Geometry check sheet. Reference: drawing and pictorial views, mm from the part's lowest x, y, z. Round coordinates to 2 decimals unless told otherwise and drop trailing zeros. Loops run counter-clockwise (first coordinate to the right, second up) from the corner with the lowest first, then second, coordinate; pieces in that order, holes last. Notation, with made-up numbers: (22, -19.5) -> (48, -19.5) arc R33 ccw to (48, 14.5) -> close; hole circle Ø8 at (16, 51). An arc over 180 degrees is marked (long way). Use one line per item in the form item = value. Start each with the question number.
(1) Material ranges on probe 1 along Y at (x, z) = (150, 17.75); probe 2 along X at (y, z) = (51.5, 20.75); probe 3 along X at (y, z) = (33.5, 17), recorded low to high. Write a range as [from, to].
(2) Sectioned sample at A-A (y = 50). Record the cut outline in (x, z), and give its area (3 significant figures).
(3) Draft check along X on the marked faces 1, 2 and 3. Enter one of: released by +X, released by -X, zero draft, split by the parting line, or undercut.
(4) Go/stop test with a flat-tipped pin: pin 1 (1 mm diameter, centred on y = 88, z = 22.5, fed in from -X). Record where the tip stops, or that it passes through.
(5) Sectioned sample at C-C (z = 21). Record the cut outline in (x, y), and give its area (3 significant figures).
(6) Sectioned sample at B-B (x = 150). Record the cut outline in (y, z).
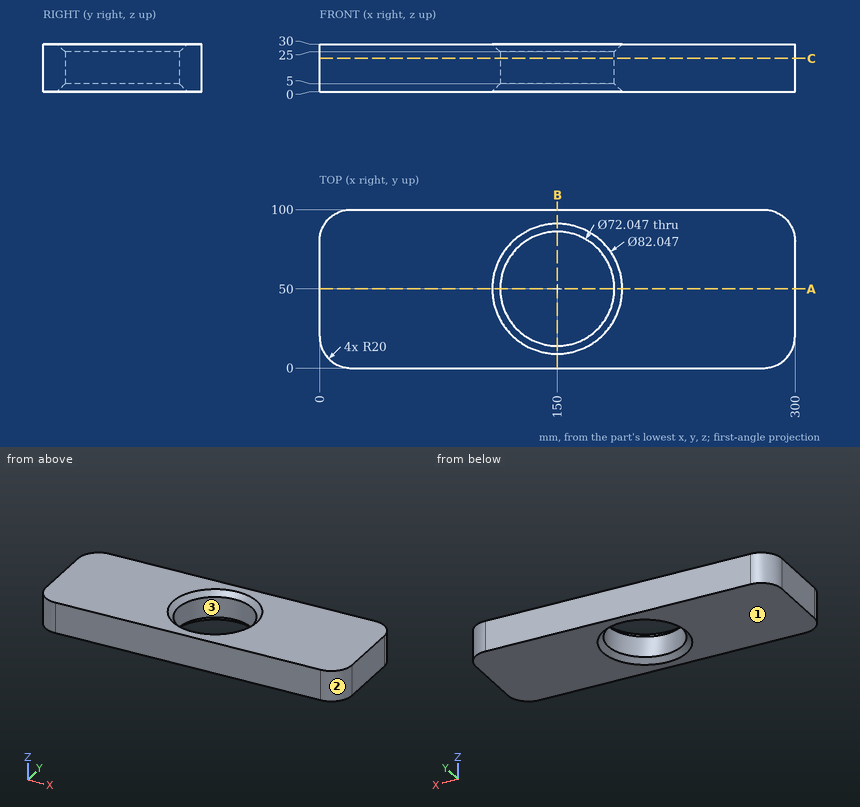
Checks:
q1.probe_1 = [0, 13.98], [86.02, 100]
q1.probe_2 = [0, 114.01], [185.99, 300]
q1.probe_3 = [0, 117.98], [182.02, 300]
q2.outline = (0, 0) -> (108.98, 0) -> (113.98, 5) -> (113.98, 25) -> (108.98, 30) -> (0, 30) -> close; (186.02, 5) -> (191.02, 0) -> (300, 0) -> (300, 30) -> (191.02, 30) -> (186.02, 25) -> close
q2.area = 6,790 mm2
q3.face_1 = zero draft
q3.face_2 = released by +X
q3.face_3 = undercut
q4.pin_1 = 1.46
q5.outline = (0, 20) arc R20 ccw to (20, 0) -> (280, 0) arc R20 ccw to (300, 20) -> (300, 80) arc R20 ccw to (280, 100) -> (20, 100) arc R20 ccw to (0, 80) -> close; hole circle Ø72.05 at (150, 50)
q5.area = 25,600 mm2
q6.outline = (0, 0) -> (8.98, 0) -> (13.98, 5) -> (13.98, 25) -> (8.98, 30) -> (0, 30) -> close; (86.02, 5) -> (91.02, 0) -> (100, 0) -> (100, 30) -> (91.02, 30) -> (86.02, 25) -> close
